from build123d import *

# Parameters (mm, degrees)
BOSS_EXTRUDE1_DEPTH       = 10
SKETCH2_R                 = 4
CUT_EXTRUDE1_DEPTH        = 4.5
SKETCH3_R                 = 2.25
CUT_EXTRUDE2_DEPTH        = 9.5
M4X0_7_TAPPED_HOLE1_D     = 3.3
M4X0_7_TAPPED_HOLE1_DEPTH = 8
M4X0_7_TAPPED_HOLE1_TIP   = 0.991420021


with BuildPart() as part:
    # Sketch1 → Boss-Extrude1 (new body)
    with BuildSketch(Plane.XY):
        Polygon((-7.612, 62.794), (1.388, 62.794), (1.388, 32.794), (5.388, 32.794), (5.388, -37.206), (-9.612, -37.206), (-9.612, 27.794), (-7.612, 27.794), align=None)
    extrude(amount=BOSS_EXTRUDE1_DEPTH)

    # Sketch2 → Cut-Extrude1 (cut)
    with BuildSketch(Plane.ZY.offset(7.612)):
        with Locations((5, 57.794)):
            Circle(SKETCH2_R)
        with Locations((5, 37.794)):
            Circle(SKETCH2_R)
    extrude(amount=-CUT_EXTRUDE1_DEPTH, mode=Mode.SUBTRACT)

    # Sketch3 → Cut-Extrude2 (cut, through all)
    with BuildSketch(Plane.ZY.offset(3.112)):
        with Locations((5, 37.794)):
            Circle(SKETCH3_R)
        with Locations((5, 57.794)):
            Circle(SKETCH3_R)
    extrude(amount=-CUT_EXTRUDE2_DEPTH, mode=Mode.SUBTRACT)

    # M4x0.7 Tapped Hole1
    with Locations(Plane.ZY.offset(9.612)):
        with Locations((5, 2.794), (5, -27.206)):
            Hole(M4X0_7_TAPPED_HOLE1_D / 2, depth=M4X0_7_TAPPED_HOLE1_DEPTH)
            with Locations((0, 0, -(M4X0_7_TAPPED_HOLE1_DEPTH + M4X0_7_TAPPED_HOLE1_TIP / 2))):  # 118° drill point
                Cone(0, M4X0_7_TAPPED_HOLE1_D / 2, M4X0_7_TAPPED_HOLE1_TIP, mode=Mode.SUBTRACT)


solid = part.part
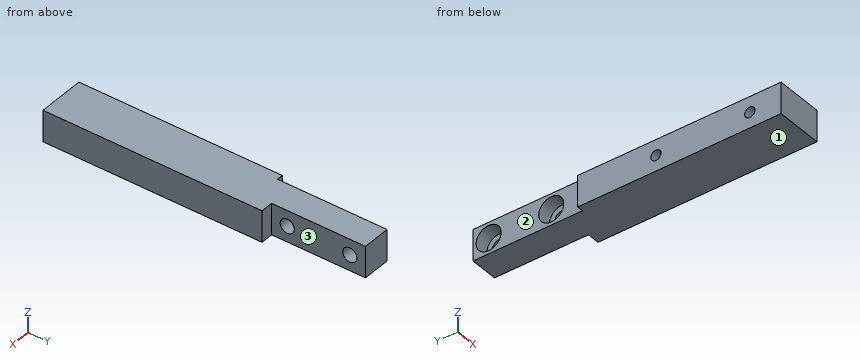
Build history of the part. All positions in model axes, mm. Face numbers are marked on the shaded views. A direction names the side the tool comes from. Give positions to 0.01 mm unless a question says otherwise; leave off trailing zeros. Order: outer loops, then holes, each group sorted by start corner. A loop starts at its lowest first (then second) coordinate and runs counter-clockwise, first axis right, second up. Notation, with made-up numbers: M 57.5,85.5 L 74.5,85.5 A27 ccw 74.5,111.5 Z; hole C -24.5,-16.5 d1. An arc over 180 degrees is marked long. Put each result on its own line as item: value.
Item 1: 3-axis set-ups, long thin cutter, end or side, ignore diameter. For the marked faces 1, 2 and 3: which of +Z, -Z, +X, -X, +Y, -Y reach the whole face in a straight line?
From the geometry:
face 1: -Z, +X, -X, +Y, -Y
face 2: +Z, -Z, -X, +Y
face 3: +Z, -Z, +X, +Y
Item 2: Flat gauge pins, fed straight in: pin 1 Ø5 at (y, z) = (44.5, 6.5) entering from +X; pin 2 Ø2 at (x, z) = (3, 3) entering from +Y; pin 3 Ø1 at (y, z) = (52, 5) entering from -X; pin 4 Ø3 at (x, y) = (-4.5, 20.5) entering from -Z. Where does each tip first touch, or does it go through?
From the geometry:
pin 1: stops at x = 1.39
pin 2: stops at y = 32.79
pin 3: stops at x = -7.61
pin 4: stops at z = 0
Item 3: Slice it at A-A, the plane x = -6.75. Write the cut outline in (y, z).
From the geometry:
outline: M -37.21,0 L 62.79,0 L 62.79,10 L -37.21,10 Z; hole C -27.21,5 d3.3; hole C 2.79,5 d3.3; hole C 37.79,5 d8; hole C 57.79,5 d8
Item 4: Probe line 1 (Y direction, x = -4.55, z = 5); line 2 (Y direction, x = -2.25, z = 4.5); line 3 (Y direction, x = 0, z = 6.5). List the from-to ranges inside material, lowest first. Write a range as [from, to].
From the geometry:
line 1: y = [-37.21, -28.86], [-25.56, 1.14], [4.44, 33.79], [41.79, 53.79], [61.79, 62.79]
line 2: y = [-37.21, -28.78], [-25.63, 1.22], [4.37, 35.6], [39.99, 55.6], [59.99, 62.79]
line 3: y = [-37.21, 36.12], [39.47, 56.12], [59.47, 62.79]
